Build history of the part. All positions in model axes, mm. A direction names the side the tool comes from. Give positions to 0.01 mm unless a question says otherwise; leave off trailing zeros. Loops run counter-clockwise (first coordinate to the right, second up) from the corner with the lowest first, then second, coordinate; pieces in that order, holes last. Notation, with made-up numbers: (37, 76.25) -> (64, 76.25) arc R17 cw to (64, 81.25) -> close; hole circle Ø3 at (88, 58.5). An arc over 180 degrees is marked (long way). Answer in a Markdown table with one row per item. Add a question column.
from build123d import *

# Parameters (mm, degrees)
CUT_EXTRUDE1_DEPTH = 10


with BuildPart() as part:
    # Sketch1 → Revolve1 (revolve)
    with BuildSketch(Plane(origin=(0, 0, 0), x_dir=(0, 0, -1), z_dir=(1, 0, 0))):
        with BuildLine():
            Line((0, 0), (0, 16.5))
            ThreePointArc((0, 16.5), (-1.148517206, 16.147528677), (-2, 15.3))
            Line((-2, 15.3), (-3, 15.3))
            Line((-3, 15.3), (-3, 14.8))
            Line((-3, 14.8), (-1, 14.8))
            Line((-1, 14.8), (-1, 0.769364806))
            Line((-1, 0.769364806), (0, 0))
        make_face()
    revolve(axis=Axis((0, 0, 0), (0, 1, 0)))

    # Sketch2 → Cut-Extrude1 (cut)
    with BuildSketch(Plane(origin=(0, 15.3, 0), x_dir=(1, 0, 0), z_dir=(0, 1, 0))):
        Polygon((0.277999407, -1.686950947), (-0.277999407, -1.686950947), (-0.277999407, -0.28662128), (-1.73927004, -0.28662128), (-1.73927004, 0.28662128), (-0.277999407, 0.28662128), (-0.277999407, 1.686950947), (0.277999407, 1.686950947), (0.277999407, 0.28662128), (1.73927004, 0.28662128), (1.73927004, -0.28662128), (0.277999407, -0.28662128), align=None)
    extrude(amount=CUT_EXTRUDE1_DEPTH, mode=Mode.SUBTRACT)


solid = part.part
(1) Saw through at A-A, the plane y = 1.75. List the corners of the cut face in (x, z), then the cut area to 3 significant figures.
(2) Wall check: line 1 along Y through (x, z) = (-0.3, 2.4); line 2 along Y through (x, z) = (1.3, 1.05); line 3 along Z through (x, y) = (0.85, 8.5). Give the ranges that are in metal, low to high. Write a range as from..to.
(3) Saw through at B-B, the plane z = 2.2. List the corners of the cut face in (x, y).
(4) 3-axis set-ups, long thin cutter, end or side, ignore diameter. For faces 1 (the flat face through (1, 14.8, -1)), 2 (the flat face through (0.278, 16, 1)): which of +Z, -Z, +X, -X, +Y, -Y reach the whole face in a straight line?
(5) Two-plate mould, pull along X, no slides. Class faces 3 (the flat face through (0, 15.3, 0)), 4 (the cylindrical face through (0, 15, -3)), 5 (the flat face through (-2, 15.3, -1)): released by +X, released by -X, zero draft, split by the parting line, or undercut.
(6) Saw through at C-C, the plane x = -2.2. List the corners of the cut face in (y, z), then the cut area to 3 significant figures.
(7) Flat gauge pins, fed straight in: pin 1 Ø3 at (y, z) = (10, 0.5) entering from -X; pin 2 Ø1.3 at (x, y) = (-1, 16) entering from -Z; pin 3 Ø1.5 at (x, z) = (0, 2) entering from +Y. Where does each tip first touch, or does it go through?
Worked answers:
| question | item | result |
|---|---|---|
| 1 | outline | circle Ø2 at (0, 0) |
| 1 | area | 3.14 mm^2 |
| 2 | line 1 | 14.8..15.3 |
| 2 | line 2 | 14.8..15.73 |
| 2 | line 3 | -0.53..0.53 |
| 3 | outline | (-2.04, 14.8) -> (2.04, 14.8) -> (2.04, 15.3) -> (-2.04, 15.3) -> close |
| 4 | face 1 | -Y |
| 4 | face 2 | +Y |
| 5 | face 3 | undercut |
| 5 | face 4 | split by the parting line |
| 5 | face 5 | zero draft |
| 6 | outline | (14.8, -2.04) -> (15.3, -2.04) -> (15.3, 2.04) -> (14.8, 2.04) -> close |
| 6 | area | 2.04 mm^2 |
| 7 | pin 1 | x = -1 |
| 7 | pin 2 | z = -1.79 |
| 7 | pin 3 | y = 16.03 |
